Answer from the drawing. Dimensions are ordinates in mm from the lowest x, y and z of the part. A direction names the side the tool comes from. Coordinates: 2 decimals unless noted, no trailing zeros. Order: outer loops, then holes, each group sorted by start corner. A loop starts at its lowest first (then second) coordinate and runs counter-clockwise, first axis right, second up. Notation, with made-up numbers: M 11,45 L 17,45 A28 ccw 17,83 Z; hole C 53.25,14 d4. An arc over 180 degrees is marked long. Use a Markdown table: item, result.
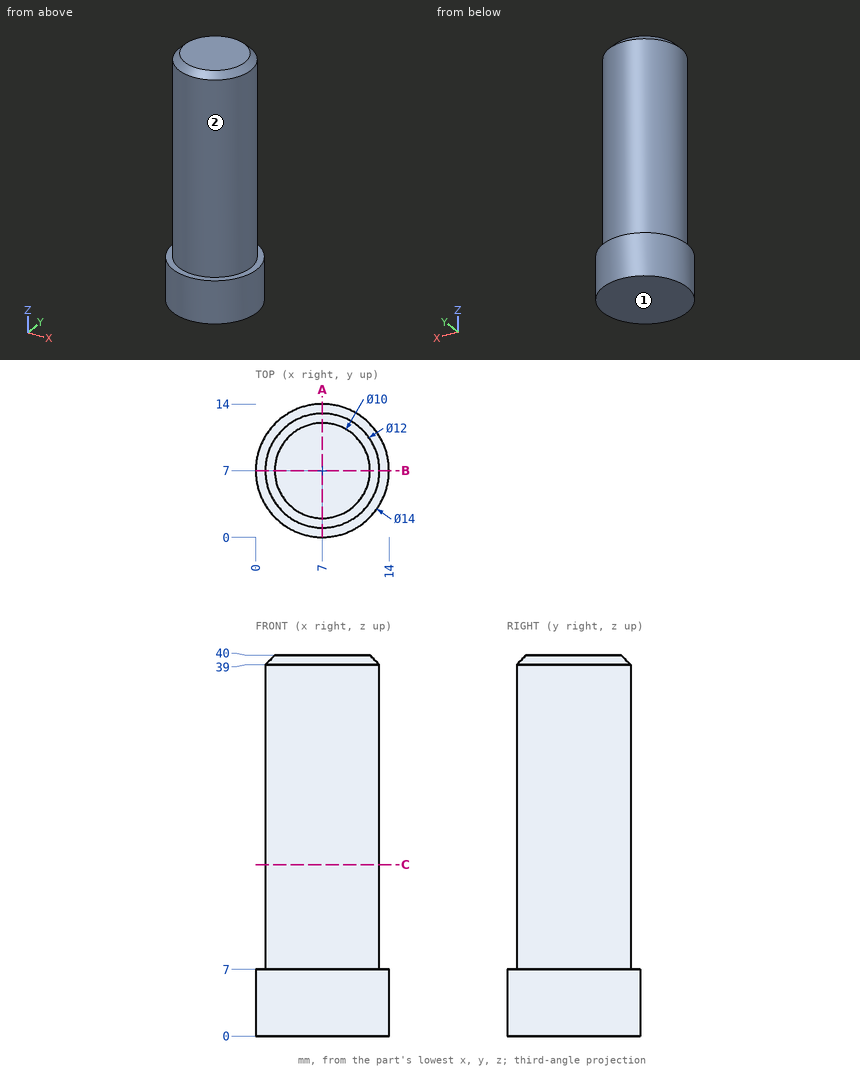
(1) Which of the six approach directions +Z, -Z, +X, -X, +Y, -Y give full straight-line access (tool end or side, diameter ignored) to the marked faces 1 and 2?
Conclusion:
| item | result |
|---|---|
| face 1 | -Z, +X, -X, +Y, -Y |
| face 2 | +Z |
(2) Given P1, Ø8, axis at y = 10.5, z = 35.5, coming from the -X side; P2, Ø2, axis at y = 6.5, z = 35.5, coming from the +X side; P3, Ø1, axis at x = 5, z = 27, coming from the -Y side, each flat-ended and moving along its own axis, determine where each tip first touches the part or whether it passes through.
Conclusion:
| item | result |
|---|---|
| P1 | x = 1 |
| P2 | x = 13 |
| P3 | y = 1.19 |
(3) A cutting plane is placed at A-A (x = 7). Determine the outline of the cut face in (y, z), then the cut area to 3 significant figures.
Conclusion:
| item | result |
|---|---|
| outline | M 0,0 L 14,0 L 14,7 L 13,7 L 13,39 L 12,40 L 2,40 L 1,39 L 1,7 L 0,7 Z |
| area | 493 mm2 |
(4) Straight lines are drawn through the part: L1, parallel to Y at x = 7, z = 17; L2, parallel to Y at x = 4, z = 14; L3, parallel to X at y = 10.25, z = 16. For each, find the intervals that lie inside material, in ascending order.
Conclusion:
| item | result |
|---|---|
| L1 | 1 to 13 |
| L2 | 1.8 to 12.2 |
| L3 | 1.96 to 12.04 |
(5) A cutting plane is placed at C-C (z = 18). Determine the outline of the cut face in (x, y).
Conclusion:
| item | result |
|---|---|
| outline | C 7,7 d12 |
